from build123d import *

# Parameters (mm, degrees)
SKETCH_1_W               = 132.5
SKETCH_1_H               = 16
SKETCH_1_R               = 2
EXTRUDE_1_DEPTH          = 4.5
FILLET_1_R               = 1
SKETCH_5_W               = 124.5
SKETCH_5_H               = 16
EXTRUDE_2_DEPTH          = 4.5
SKETCH_6_W               = 120
SKETCH_6_H               = 5
EXTRUDE_3_DEPTH          = 4
CUT_EXTRUDE_1_DEPTH      = 74.186832832
CUT_EXTRUDE_1_DEPTH_BACK = 74.186832832
SKETCH_2_R               = 1.65
FILLET_3_R               = 2


with BuildPart() as part:
    # Sketch 1 → Extrude 1 (new body)
    # profile 1 of 5: a face of its own
    with BuildSketch(Plane.XY):
        Rectangle(SKETCH_1_W, SKETCH_1_H)
    # profile 2 of 5: a face of its own
    with BuildSketch(Plane.XY):
        with BuildLine():
            Line((-66.25, 8), (-69.25, 8))
            ThreePointArc((-69.25, 8), (-72.25, 5), (-69.25, 2))
            Line((-69.25, 2), (-66.25, 2))
            Line((-66.25, 2), (-66.25, 8))
        make_face()
        with Locations((-69.25, 5)):
            Circle(SKETCH_1_R, mode=Mode.SUBTRACT)
    # profile 3 of 5: a face of its own
    with BuildSketch(Plane.XY):
        with BuildLine():
            Line((-66.25, -8), (-66.25, -2))
            Line((-66.25, -2), (-69.25, -2))
            ThreePointArc((-69.25, -2), (-72.25, -5), (-69.25, -8))
            Line((-69.25, -8), (-66.25, -8))
        make_face()
        with Locations((-69.25, -5)):
            Circle(SKETCH_1_R, mode=Mode.SUBTRACT)
    # profile 4 of 5: a face of its own
    with BuildSketch(Plane.XY):
        with BuildLine():
            Line((69.25, 8), (66.25, 8))
            Line((66.25, 8), (66.25, 2))
            Line((66.25, 2), (69.25, 2))
            ThreePointArc((69.25, 2), (72.25, 5), (69.25, 8))
        make_face()
        with Locations((69.25, 5)):
            Circle(SKETCH_1_R, mode=Mode.SUBTRACT)
    # profile 5 of 5: a face of its own
    with BuildSketch(Plane.XY):
        with BuildLine():
            Line((69.25, -2), (66.25, -2))
            Line((66.25, -2), (66.25, -8))
            Line((66.25, -8), (69.25, -8))
            ThreePointArc((69.25, -8), (72.25, -5), (69.25, -2))
        make_face()
        with Locations((69.25, -5)):
            Circle(SKETCH_1_R, mode=Mode.SUBTRACT)
    extrude(amount=EXTRUDE_1_DEPTH)

    # Fillet 1
    fillet_1_edges = [part.edges().sort_by_distance(p)[0] for p in [
        (-66.25, -2, 2.25),
        (-66.25, 2, 2.25),
        (66.25, 2, 2.25),
        (66.25, -2, 2.25),
    ]]
    fillet(fillet_1_edges, radius=FILLET_1_R)

    # Sketch 5 → Extrude 2 (add)
    with BuildSketch(Plane.XY.offset(4.5)):
        Rectangle(SKETCH_5_W, SKETCH_5_H)
    extrude(amount=EXTRUDE_2_DEPTH)

    # Sketch 6 → Extrude 3 (add)
    with BuildSketch(Plane.XY.offset(9)):
        Rectangle(SKETCH_6_W, SKETCH_6_H)
    extrude(amount=EXTRUDE_3_DEPTH)

    # Sketch 2 → Cut-Extrude 1 (cut, two sides: drawn at the far end of the back side and taken through both)
    with BuildSketch(Plane.XY.offset(4.5).offset(-CUT_EXTRUDE_1_DEPTH_BACK)):
        with Locations((35, 0)):
            Circle(SKETCH_2_R)
        with Locations((20, 0)):
            Circle(SKETCH_2_R)
        with Locations(Location((-20, 0, 0), (0, 0, 180))):
            Circle(SKETCH_2_R)
        with Locations(Location((-35, 0, 0), (0, 0, 180))):
            Circle(SKETCH_2_R)
    extrude(amount=CUT_EXTRUDE_1_DEPTH + CUT_EXTRUDE_1_DEPTH_BACK, mode=Mode.SUBTRACT)

    # Fillet 3
    fillet_3_edges = [part.edges().sort_by_distance(p)[0] for p in [
        (-60, 2.5, 11),
        (-60, -2.5, 11),
        (60, -2.5, 11),
        (60, 2.5, 11),
        (-62.25, 8, 6.75),
        (-62.25, -8, 6.75),
        (62.25, -8, 6.75),
        (62.25, 8, 6.75),
    ]]
    fillet(fillet_3_edges, radius=FILLET_3_R)


solid = part.part
Can you work these out from the model? Positions are in its coordinate system, mm. A direction names the side the tool comes from. Give positions to 0.01 mm unless a question says otherwise; leave off trailing zeros. Loops run counter-clockwise (first coordinate to the right, second up) from the corner with the lowest first, then second, coordinate; pieces in that order, holes last. Notation, with made-up numbers: (75, -16) -> (86, -16) arc R20 ccw to (86, 0) -> close; hole circle Ø11 at (-39.5, 45.25). An arc over 180 degrees is marked (long way). Write item = value, one per line.
1) For faces 4 (the flat face through (62.25, 0, 7)), 5 (the flat face through (-62.25, 0, 7)), 6 (the flat face through (-1, 2.5, 11)), 7 (the flat face through (-1, -2.5, 11)), which set-ups out of +Z, -Z, +X, -X, +Y, -Y let a thin tool reach every point of the face, with its end or its side?
Check result:
face_4 = +Z, +X, +Y, -Y
face_5 = +Z, -X, +Y, -Y
face_6 = +Z, +X, -X, +Y
face_7 = +Z, +X, -X, -Y
2) Thinking about a two-plate mould opening in X: for faces 1 (the flat face through (-1, 0, 0)), 2 (the cylindrical face through (18.69, -1, 6.41)), 3 (the cylindrical face through (-72.25, -4.93, 2.22)), which applies, released by +X, released by -X, zero draft, split by the parting line, or undercut?
Check result:
face_1 = zero draft
face_2 = undercut
face_3 = released by -X
3) Will these pins go through, and if not, where does the flat tip stop? pin 1 (2 mm diameter, centred on y = -3, z = 6.5, fed in from +X); pin 2 (2 mm diameter, centred on x = -20, y = 0, fed in from -Z); pin 3 (0.6 mm diameter, centred on y = 0, z = 3, fed in from -X); pin 4 (2 mm diameter, centred on x = -15.5, z = 10.5, fed in from +Y).
Check result:
pin_1 = 62.25
pin_2 = through
pin_3 = -66.25
pin_4 = 2.5
4) Suppose I cut it at B-B on z = 3.25. Give the number of separate pieces and of enclosed holes in the cut face, then the cut area to 3 significant figures.
Check result:
separate_pieces = 1
enclosed_holes = 8
area = 2,160 mm2
5) Suppose I cut it at C-C on x = 10. Write out the boundary of the cut face in (y, z).
Check result:
outline = (-8, 0) -> (8, 0) -> (8, 9) -> (2.5, 9) -> (2.5, 13) -> (-2.5, 13) -> (-2.5, 9) -> (-8, 9) -> close
6) Suppose I cut it at A-A on x = 35. Write out the boundary of the cut face in (y, z).
Check result:
outline = (-8, 0) -> (-1.65, 0) -> (-1.65, 13) -> (-2.5, 13) -> (-2.5, 9) -> (-8, 9) -> close; (1.65, 0) -> (8, 0) -> (8, 9) -> (2.5, 9) -> (2.5, 13) -> (1.65, 13) -> close
7) I need wall thicknesses on L1, parallel to Y at x = -69.25, z = 3.3; L2, parallel to X at y = 0.25, z = 12; L3, parallel to Y at x = -35, z = 7.75. Which ranges of each line are inside material? Lowest first, please. Write a range as from..to.
Check result:
L1 = -8..-7, -3..-2, 2..3, 7..8
L2 = -60..-36.63, -33.37..-21.63, -18.37..18.37, 21.63..33.37, 36.63..60
L3 = -8..-1.65, 1.65..8
